For this review, take the finished solid that the model builds, in its own axes (mm). A direction names the side the tool comes from. Round coordinates to 2 decimals unless told otherwise and drop trailing zeros. Loops run counter-clockwise (first coordinate to the right, second up) from the corner with the lowest first, then second, coordinate; pieces in that order, holes last. Notation, with made-up numbers: (36.25, 17) -> (50.25, 17) arc R17 cw to (50.25, 46) -> close; hole circle Ø6 at (-7.75, -12.75). An arc over 180 degrees is marked (long way). Use one line per item in the form item = value. Start each with the question number.
from build123d import *

# Parameters (mm, degrees)
BOSS_EXTRUDE1_DEPTH          = 5
ARDUINO_UNO_HOLES_D          = 2.5
L298N_HOLES_D                = 2.5
PROTOBOARD_HOLES_D           = 2.5
L_BRACKET_HOLES_D            = 3.3
POWER_BLOCK_SLOTS_DEPTH      = 126.099960032
CABLE_MANAGEMENT_SLOTS_DEPTH = 126.099960032
CUT_EXTRUDE3_START           = -10
CUT_EXTRUDE3_DEPTH           = 10
WALL_MOUNTING_HOLES_D        = 6.35


with BuildPart() as part:
    # Sketch1 → Boss-Extrude1 (new body)
    with BuildSketch(Plane(origin=(0, 0, 0), x_dir=(1, 0, 0), z_dir=(0, 1, 0))):
        with BuildLine():
            Line((-90, -75), (90, -75))
            ThreePointArc((90, -75), (97.071067812, -72.071067812), (100, -65))
            Line((100, -65), (100, 65))
            ThreePointArc((100, 65), (97.071067812, 72.071067812), (90, 75))
            Line((90, 75), (-90, 75))
            ThreePointArc((-90, 75), (-97.071067812, 72.071067812), (-100, 65))
            Line((-100, 65), (-100, -65))
            ThreePointArc((-100, -65), (-97.071067812, -72.071067812), (-90, -75))
        make_face()
    extrude(amount=BOSS_EXTRUDE1_DEPTH)

    # arduino uno holes (through all)
    with Locations(Plane(origin=(0, 5, 0), x_dir=(1, 0, 0), z_dir=(0, 1, 0))):
        with Locations((27.1, -27), (27.1, -54.9), (-23.7, -11.8), (-25, -60)):
            Hole(ARDUINO_UNO_HOLES_D / 2)

    # l298n holes (through all)
    with Locations(Plane(origin=(0, 5, 0), x_dir=(1, 0, 0), z_dir=(0, 1, 0))):
        with Locations((52.7, -45), (90, -45), (90, -7.7), (52.7, -7.7)):
            Hole(L298N_HOLES_D / 2)

    # protoboard holes (through all)
    with Locations(Plane(origin=(0, 5, 0), x_dir=(1, 0, 0), z_dir=(0, 1, 0))):
        with Locations((-50, 21), (14, 21), (14, 65), (-50, 65)):
            Hole(PROTOBOARD_HOLES_D / 2)

    # l-bracket holes (through all)
    with Locations(Plane(origin=(0, 5, 0), x_dir=(1, 0, 0), z_dir=(0, 1, 0))):
        with Locations((61, 55), (90, 55), (90, 25), (61, 25)):
            Hole(L_BRACKET_HOLES_D / 2)

    # Sketch24 → power block slots (cut, through all)
    with BuildSketch(Plane(origin=(0, 5, 0), x_dir=(1, 0, 0), z_dir=(0, 1, 0))):
        with BuildLine():
            Line((-60, -35), (-90, -35))
            ThreePointArc((-90, -35), (-95, -30), (-90, -25))
            Line((-90, -25), (-60, -25))
            ThreePointArc((-60, -25), (-55, -30), (-60, -35))
        make_face()
        with BuildLine():
            Line((-60, -45), (-90, -45))
            ThreePointArc((-90, -45), (-95, -50), (-90, -55))
            Line((-90, -55), (-60, -55))
            ThreePointArc((-60, -55), (-55, -50), (-60, -45))
        make_face()
    extrude(amount=-POWER_BLOCK_SLOTS_DEPTH, mode=Mode.SUBTRACT)

    # Sketch26 → cable management slots (cut, through all)
    with BuildSketch(Plane(origin=(0, 5, 0), x_dir=(1, 0, 0), z_dir=(0, 1, 0))):
        with BuildLine():
            Line((-50, 14), (14, 14))
            ThreePointArc((14, 14), (16.5, 11.5), (14, 9))
            Line((14, 9), (-50, 9))
            ThreePointArc((-50, 9), (-52.5, 11.5), (-50, 14))
        make_face()
        with BuildLine():
            Line((26, 65), (26, 21))
            ThreePointArc((26, 21), (23.5, 18.5), (21, 21))
            Line((21, 21), (21, 65))
            ThreePointArc((21, 65), (23.5, 67.5), (26, 65))
        make_face()
        with BuildLine():
            Line((68.5, 57), (82.5, 57))
            ThreePointArc((82.5, 57), (84.5, 55), (82.5, 53))
            Line((82.5, 53), (68.5, 53))
            ThreePointArc((68.5, 53), (66.5, 55), (68.5, 57))
        make_face()
        with BuildLine():
            Line((68.5, 27), (82.5, 27))
            ThreePointArc((82.5, 27), (84.5, 25), (82.5, 23))
            Line((82.5, 23), (68.5, 23))
            ThreePointArc((68.5, 23), (66.5, 25), (68.5, 27))
        make_face()
        with BuildLine():
            Line((52.7, 4.3), (90, 4.3))
            ThreePointArc((90, 4.3), (92.5, 1.8), (90, -0.7))
            Line((90, -0.7), (52.7, -0.7))
            ThreePointArc((52.7, -0.7), (50.2, 1.8), (52.7, 4.3))
        make_face()
        with BuildLine():
            Line((45.7, -7.7), (45.7, -45))
            ThreePointArc((45.7, -45), (43.2, -47.5), (40.7, -45))
            Line((40.7, -45), (40.7, -7.7))
            ThreePointArc((40.7, -7.7), (43.2, -5.2), (45.7, -7.7))
        make_face()
        with BuildLine():
            Line((-25, -67), (27.1, -67))
            ThreePointArc((27.1, -67), (29.6, -69.5), (27.1, -72))
            Line((27.1, -72), (-25, -72))
            ThreePointArc((-25, -72), (-27.5, -69.5), (-25, -67))
        make_face()
        with BuildLine():
            Line((-43, -30), (-43, -50))
            ThreePointArc((-43, -50), (-45.5, -52.5), (-48, -50))
            Line((-48, -50), (-48, -30))
            ThreePointArc((-48, -30), (-45.5, -27.5), (-43, -30))
        make_face()
        with BuildLine():
            Line((-23.7, 0.2), (27.1, 0.2))
            ThreePointArc((27.1, 0.2), (29.6, -2.3), (27.1, -4.8))
            Line((27.1, -4.8), (-23.7, -4.8))
            ThreePointArc((-23.7, -4.8), (-26.2, -2.3), (-23.7, 0.2))
        make_face()
        with BuildLine():
            Line((-57, 65), (-57, 21))
            ThreePointArc((-57, 21), (-59.5, 18.5), (-62, 21))
            Line((-62, 21), (-62, 65))
            ThreePointArc((-62, 65), (-59.5, 67.5), (-57, 65))
        make_face()
        with BuildLine():
            Line((90, -57), (52.7, -57))
            ThreePointArc((52.7, -57), (50.2, -54.5), (52.7, -52))
            Line((52.7, -52), (90, -52))
            ThreePointArc((90, -52), (92.5, -54.5), (90, -57))
        make_face()
    extrude(amount=-CABLE_MANAGEMENT_SLOTS_DEPTH, mode=Mode.SUBTRACT)

    # Sketch27 → Cut-Extrude3 (cut)
    with BuildSketch(Plane(origin=(0, 5, 0), x_dir=(1, 0, 0), z_dir=(0, 1, 0)).offset(CUT_EXTRUDE3_START)):
        with BuildLine():
            Line((-69.5, -10), (-69.5, 65))
            ThreePointArc((-69.5, 65), (-66.571067812, 72.071067812), (-59.5, 75))
            Line((-59.5, 75), (-90, 75))
            ThreePointArc((-90, 75), (-97.071067812, 72.071067812), (-100, 65))
            Line((-100, 65), (-100, -30))
            ThreePointArc((-100, -30), (-97.071067812, -22.928932188), (-90, -20))
            Line((-90, -20), (-79.5, -20))
            ThreePointArc((-79.5, -20), (-72.428932188, -17.071067812), (-69.5, -10))
        make_face()
    extrude(amount=CUT_EXTRUDE3_DEPTH, mode=Mode.SUBTRACT)

    # wall-mounting holes (through all)
    with Locations(Plane(origin=(0, 5, 0), x_dir=(1, 0, 0), z_dir=(0, 1, 0))):
        with Locations((-90, -65), (90, -65), (39.784709297, 65), (-52.5, -4.3)):
            Hole(WALL_MOUNTING_HOLES_D / 2)


solid = part.part
Item 1: Take a section at A-A on x = 23.5. Give the boundary of the cut face in (y, z).
Item 2: Take a section at D-D on y = 0.8. Give the number of separate pieces and of enclosed holes in the cut face, plus the area to 3 significant figures.
Item 3: Take a section at C-C on x = -45.5. Give the boundary of the cut face in (y, z).
Item 4: For P1, Ø1, axis at x = -61, y = 2.5, coming from the -Z side; P2, Ø1.5, axis at y = 3, z = -49.5, coming from the -X side, all flat-tipped, find the tip position at first contact; note any pin that passes through.
Item 5: Take a section at B-B on z = 37.5. Give the boundary of the cut face in (x, y).
Item 6: Draft analysis for pull direction X (two halves, no side actions). For faces 1 (the flat face through (-1, 0, -1)), 2 (the cylindrical face through (-72.51, 2.46, 17.15)), 3 (the flat face through (76, 3, -53)), state which applies: +X half, -X half, draft (parallel to the pull), parting line (faces both ways), or undercut.
Item 7: Machinability: for faces 4 (the flat face through (-100, 2, 47)), 5 (the flat face through (75, 3, -57)), 6 (the flat face through (-69.5, 2, -27)), which of the approach directions +Z, -Z, +X, -X, +Y, -Y give a long, thin tool a straight path to every point of the face, cutting with its end or side? Answer none if there is none.
Item 8: Wall thickness on line 1 (X direction, y = 1.4, z = 41.5); line 2 (Z direction, x = 61, y = 1.45); line 3 (X direction, y = 2.95, z = -59.5): over which ranges is each line inside the solid? List them lowest first.
Results:
q1.outline = (0, -75) -> (5, -75) -> (5, -67.5) -> (0, -67.5) -> close; (0, -18.5) -> (5, -18.5) -> (5, -0.2) -> (0, -0.2) -> close; (0, 4.8) -> (5, 4.8) -> (5, 67) -> (0, 67) -> close; (0, 72) -> (5, 72) -> (5, 75) -> (0, 75) -> close
q2.separate_pieces = 1
q2.enclosed_holes = 33
q2.area = 23,800 mm2
q3.outline = (0, -75) -> (5, -75) -> (5, -14) -> (0, -14) -> close; (0, -9) -> (5, -9) -> (5, 27.5) -> (0, 27.5) -> close; (0, 52.5) -> (5, 52.5) -> (5, 75) -> (0, 75) -> close
q4.P1 = -74.95
q4.P2 = -69.5
q5.outline = (-100, 0) -> (-48, 0) -> (-48, 5) -> (-100, 5) -> close; (-43, 0) -> (40.7, 0) -> (40.7, 5) -> (-43, 5) -> close; (45.7, 0) -> (100, 0) -> (100, 5) -> (45.7, 5) -> close
q6.face_1 = draft
q6.face_2 = -X half
q6.face_3 = undercut
q7.face_4 = +Z, -Z, -X, +Y, -Y
q7.face_5 = +Y, -Y
q7.face_6 = -Z, -X, +Y, -Y
q8.line_1 = -100 to -48, -43 to 40.7, 45.7 to 100
q8.line_2 = -75 to -56.65, -53.35 to -26.65, -23.35 to -4.3, 0.7 to 52, 57 to 75
q8.line_3 = -69.5 to -62, -57 to 21, 26 to 100
